Verification items for the finished model (mm, model axes). A direction names the side the tool comes from. Coordinates: 2 decimals unless noted, no trailing zeros. Order: outer loops, then holes, each group sorted by start corner. A loop starts at its lowest first (then second) coordinate and runs counter-clockwise, first axis right, second up. Notation, with made-up numbers: (17.25, -8) -> (28.25, -8) arc R13 ccw to (28.25, 17) -> close; hole circle Ø4 at (69.25, -8). An arc over 180 degrees is marked (long way). Write item = value, one per line. Start each with the question number.
1. Thickness scan on line 1 along X through (y, z) = (-5.5, -8); line 2 along Z through (x, y) = (0, -4.5); line 3 along X through (y, z) = (-5, 10.5). Record the ranges inside material, lowest first. Write a range as from..to.
2. Release check for a two-part mould opening along X. For faces 1 (the cylindrical face through (-7.11, -3.16, 9.2)), 2 (the flat face through (8.2, 0, 4.5)), 3 (the cylindrical face through (8.767, -3.155, -16.856)), 4 (the cylindrical face through (8.15, -3.16, 6.97)) record: +X half, -X half, draft (parallel to the pull), parting line (faces both ways), or undercut.
3. Cross-section at A-A on x = 0. Record the cut outline in (y, z), plus the area to 3 significant figures.
4. Set-up check for faces 5 (the flat face through (8.2, -6.4, 4.5)), 6 (the cylindrical face through (-9.1, -3.16, 0.16)): record each of +Z, -Z, +X, -X, +Y, -Y from which the full face is reachable in a straight line by a thin tool's end or side.
5. Cross-section at B-B on z = -12.5. Record the cut outline in (x, y).
6. Cross-section at D-D on x = 13. Record the cut outline in (y, z), plus the area to 3 significant figures.
7. Go/stop test with a flat-tipped pin: P1, Ø1.9, axis at x = -8.49, z = 8.49, coming from the -Y side. Record where the tip stops, or that it passes through.
8. Cross-section at C-C on y = -5.5. Record the cut outline in (x, z), plus the area to 3 significant figures.
from build123d import *

# Parameters (mm, degrees)
F0_R            = 19
F1_DEPTH        = 6.4
F2_R            = 1.55
F3_DEPTH        = 25.4
F3_COPIES_COUNT = 4
F4_R            = 9.1
F5_DEPTH        = 6.401
F6_R            = 3.05
F7_DEPTH        = 6.401


# Not quite as in the source:
# - a pattern or mirror of a feature is missing from the dataset's text; its kind, count and spacing are read off the source's solid


with BuildPart() as f1:
    # F0 (on Front) → F1 (new body)
    with BuildSketch(Plane.XZ):
        Circle(F0_R)
    extrude(amount=F1_DEPTH)

    # F2 (on Front) → F3 (cut)
    with BuildSketch(Plane.XZ):
        with Locations((8.4852813742, 8.4852813742)):
            Circle(F2_R)
    f3 = extrude(amount=F3_DEPTH, mode=Mode.SUBTRACT)

    # F3_copies: F3 ×4 about axis
    f3_copies_axis = Axis((0, 0, 0), (0, 1, 0))
    for i in range(1, F3_COPIES_COUNT):
        add(f3.rotate(f3_copies_axis, i * 360 / F3_COPIES_COUNT), mode=Mode.SUBTRACT)

    # F4 (on Front) → F5 (cut, through all)
    with BuildSketch(Plane.XZ):
        Circle(F4_R)
    extrude(amount=F5_DEPTH, mode=Mode.SUBTRACT)

    # F6 (on Front) → F7 (cut, through all)
    with BuildSketch(Plane.XZ):
        with Locations((0, 10.5)):
            Circle(F6_R)
        with Locations((0, -10.5)):
            Circle(F6_R)
    extrude(amount=F7_DEPTH, mode=Mode.SUBTRACT)


solid = f1.part
Worked out:
q1.line_1 = -17.23..-9.96, -7.01..-4.34, 4.34..7.01, 9.96..17.23
q1.line_2 = -19..-13.55, 13.55..19
q1.line_3 = -15.84..-3.05, 3.05..15.84
q2.face_1 = undercut
q2.face_2 = draft
q2.face_3 = parting line
q2.face_4 = undercut
q3.outline = (-6.4, -19) -> (0, -19) -> (0, -13.55) -> (-6.4, -13.55) -> close; (-6.4, 13.55) -> (0, 13.55) -> (0, 19) -> (-6.4, 19) -> close
q3.area = 69.8 mm²
q4.face_5 = +Z, -Z, +X, -X, -Y
q4.face_6 = +Y, -Y
q5.outline = (-14.31, -6.4) -> (-2.3, -6.4) -> (-2.3, 0) -> (-14.31, 0) -> close; (2.3, -6.4) -> (14.31, -6.4) -> (14.31, 0) -> (2.3, 0) -> close
q6.outline = (-6.4, -13.86) -> (0, -13.86) -> (0, 13.86) -> (-6.4, 13.86) -> close
q6.area = 177 mm²
q7.P1 = through
q8.outline = circle Ø38 at (0, 0); hole circle Ø3.1 at (-8.49, -8.49); hole circle Ø3.1 at (-8.49, 8.49); hole (-2.5, -8.75) arc R3.05 ccw (long way) to (2.5, -8.75) arc R9.1 ccw to (2.5, 8.75) arc R3.05 ccw (long way) to (-2.5, 8.75) arc R9.1 ccw to start; hole circle Ø3.1 at (8.49, -8.49); hole circle Ø3.1 at (8.49, 8.49)
q8.area = 797 mm²
